Here's the drawing with two shaded views (mm, measured from the low corner). I have some questions. Coordinates: 2 decimals unless noted, no trailing zeros. Loops run counter-clockwise (first coordinate to the right, second up) from the corner with the lowest first, then second, coordinate; pieces in that order, holes last. Notation, with made-up numbers: (-18, -33.75) -> (8, -33.75) arc R17 ccw to (8, -8.75) -> close; hole circle Ø4 at (-19, 40.25). An arc over 180 degrees is marked (long way). Answer as a JSON object with one key per item and string values. Group by question number.
1) I want a section at B-B (x = 47). Write out the boundary of the cut face in (y, z), then the cut area to 3 significant figures.
2) I'm going to push a flat-ended pin straight in: pin 1 (3.5 mm diameter, centred on x = 47, y = 49.5, fed in from -Z). Where does the tip first touch, or does it pass through?
3) I want a section at A-A (y = 10.2). Write out the boundary of the cut face in (x, z).
4) I need wall thicknesses on probe 1 along Y at (x, z) = (14, 1.05); probe 2 along Y at (x, z) = (13.5, 0.75). Which ranges of each line are inside material? Lowest first, please. Write a range as [from, to].
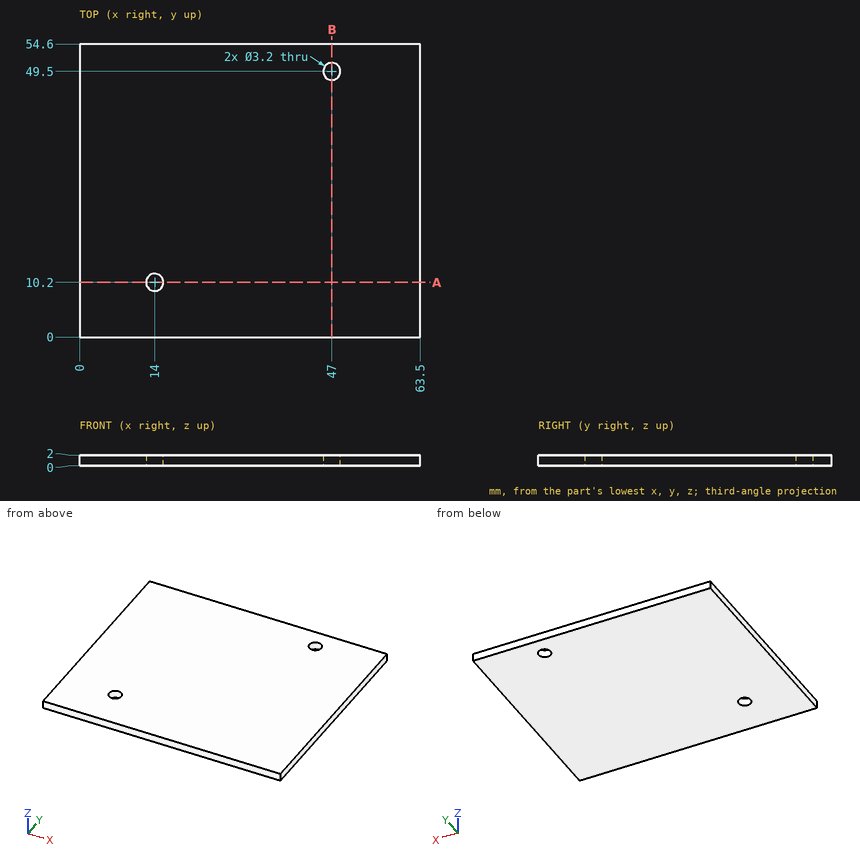
Determined:
{
 "1": {"outline": "(0, 0) -> (47.9, 0) -> (47.9, 2) -> (0, 2) -> close; (51.1, 0) -> (54.6, 0) -> (54.6, 2) -> (51.1, 2) -> close", "area": "103 mm^2"},
 "2": {"pin 1": "z = 0"},
 "3": {"outline": "(0, 0) -> (12.4, 0) -> (12.4, 2) -> (0, 2) -> close; (15.6, 0) -> (63.5, 0) -> (63.5, 2) -> (15.6, 2) -> close"},
 "4": {"probe 1": "[0, 8.6], [11.8, 54.6]", "probe 2": "[0, 8.68], [11.72, 54.6]"}
}
